Can you work these out from the drawing? Everything is in mm from the part's minimum corner. A direction names the side the tool comes from. Give positions to 0.01 mm unless a question says otherwise; leave off trailing zeros. Write each loop counter-clockwise with the first axis right and the second up, starting at its lowest first coordinate (ties: lowest second). Pieces come first, ordered by that corner, then holes. Notation, with made-up numbers: (66, 80) -> (94, 80) arc R25 cw to (94, 113) -> close; hole circle Ø4 at (12, 69.5). An arc over 180 degrees is marked (long way). Answer as CSV lines item,"result". Start each with the question number.
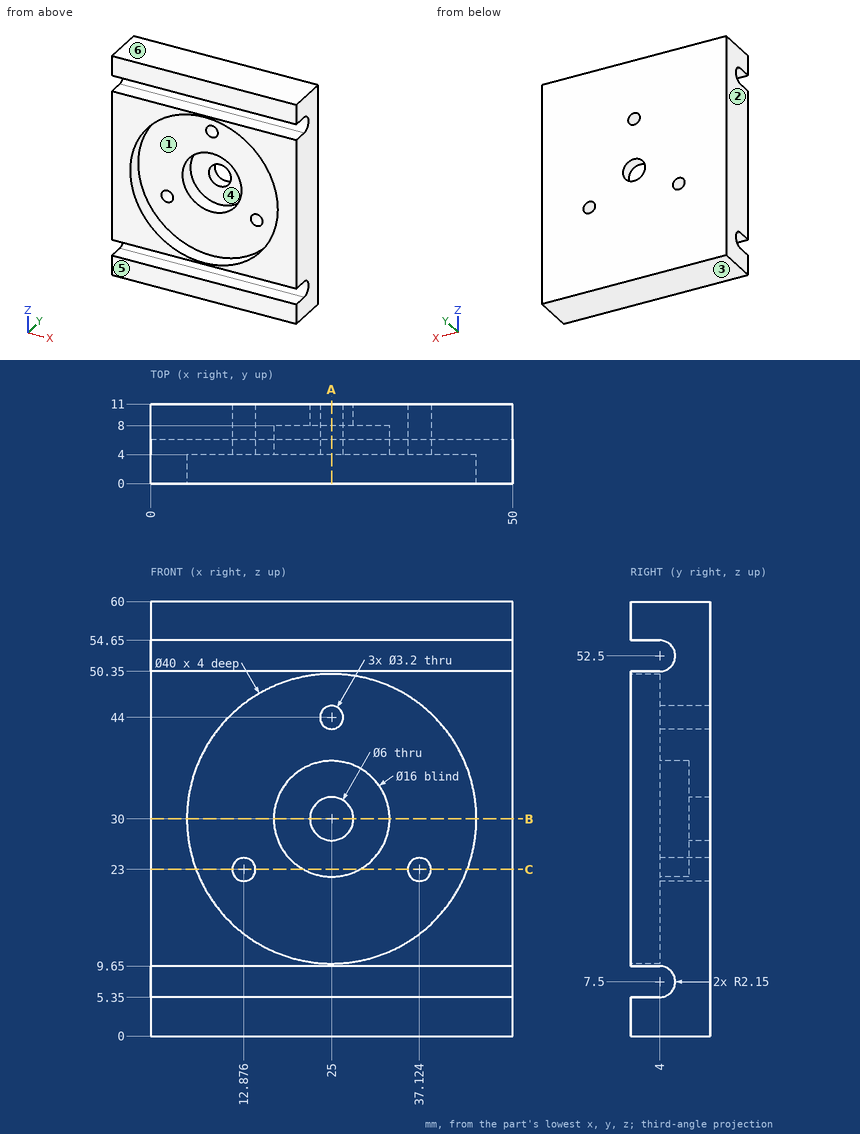
Item 1: For the marked faces 1 and 2, which set-ups out of +Z, -Z, +X, -X, +Y, -Y let a thin tool reach every point of the face, with its end or its side?
Item 2: If I drill on line 1 (Z direction, x = 25, y = 1.6); line 2 (Z direction, x = 5, y = 5.25); line 3 (Z direction, x = 43.5, y = 4.75) (1 decimal), over which ranges is the centre line in solid material (lowest first)? Write a range as [from, to].
Item 3: If we section it at B-B (z = 30): Please give me the cut outline in (x, y), and give its area (3 significant figures).
Item 4: I'm going to push flat-ended pins straight in: pin 1 (8 mm diameter, centred on x = 39, z = 33.5, fed in from -Y); pin 2 (1.9 mm diameter, centred on x = 25, z = 44, fed in from -Y); pin 3 (8 mm diameter, centred on x = 25, z = 30, fed in from -Y). Where does each tip first touch, or does it pass through?
Item 5: We'd pull the mould along Z, two halves only. Please class the marked faces 3, 4, 5 and 6: released by +Z, released by -Z, zero draft, split by the parting line, or undercut.
Item 6: If we section it at A-A (x = 25): Please give me the cut outline in (y, z), and give its area (3 significant figures).
Item 7: If we section it at C-C (z = 23): Please give me the cut outline in (x, y) (1 decimal).
Final values:
1,face 1,"-Y"
1,face 2,"+Z, -Z, -X, +Y, -Y"
2,line 1,"[0, 5.35], [9.65, 10], [50, 50.35], [54.65, 60]"
2,line 2,"[0, 5.75], [9.25, 50.75], [54.25, 60]"
2,line 3,"[0, 5.5], [9.5, 50.5], [54.5, 60]"
3,outline,"(0, 0) -> (5, 0) -> (5, 4) -> (17, 4) -> (17, 8) -> (22, 8) -> (22, 11) -> (0, 11) -> close; (28, 8) -> (33, 8) -> (33, 4) -> (45, 4) -> (45, 0) -> (50, 0) -> (50, 11) -> (28, 11) -> close"
3,area,"308 mm2"
4,pin 1,"y = 4"
4,pin 2,"through"
4,pin 3,"y = 8"
5,face 3,"released by -Z"
5,face 4,"undercut"
5,face 5,"zero draft"
5,face 6,"released by +Z"
6,outline,"(0, 0) -> (11, 0) -> (11, 27) -> (8, 27) -> (8, 22) -> (4, 22) -> (4, 10) -> (0, 10) -> (0, 9.65) -> (4, 9.65) arc R2.15 cw to (4, 5.35) -> (0, 5.35) -> close; (0, 50) -> (4, 50) -> (4, 45.6) -> (11, 45.6) -> (11, 60) -> (0, 60) -> (0, 54.65) -> (4, 54.65) arc R2.15 cw to (4, 50.35) -> (0, 50.35) -> close; (4, 38) -> (8, 38) -> (8, 33) -> (11, 33) -> (11, 42.4) -> (4, 42.4) -> close"
6,area,"347 mm2"
7,outline,"(0, 0) -> (6.3, 0) -> (6.3, 4) -> (11.3, 4) -> (11.3, 11) -> (0, 11) -> close; (14.5, 4) -> (21.1, 4) -> (21.1, 8) -> (28.9, 8) -> (28.9, 4) -> (35.5, 4) -> (35.5, 11) -> (14.5, 11) -> close; (38.7, 4) -> (43.7, 4) -> (43.7, 0) -> (50, 0) -> (50, 11) -> (38.7, 11) -> close"
